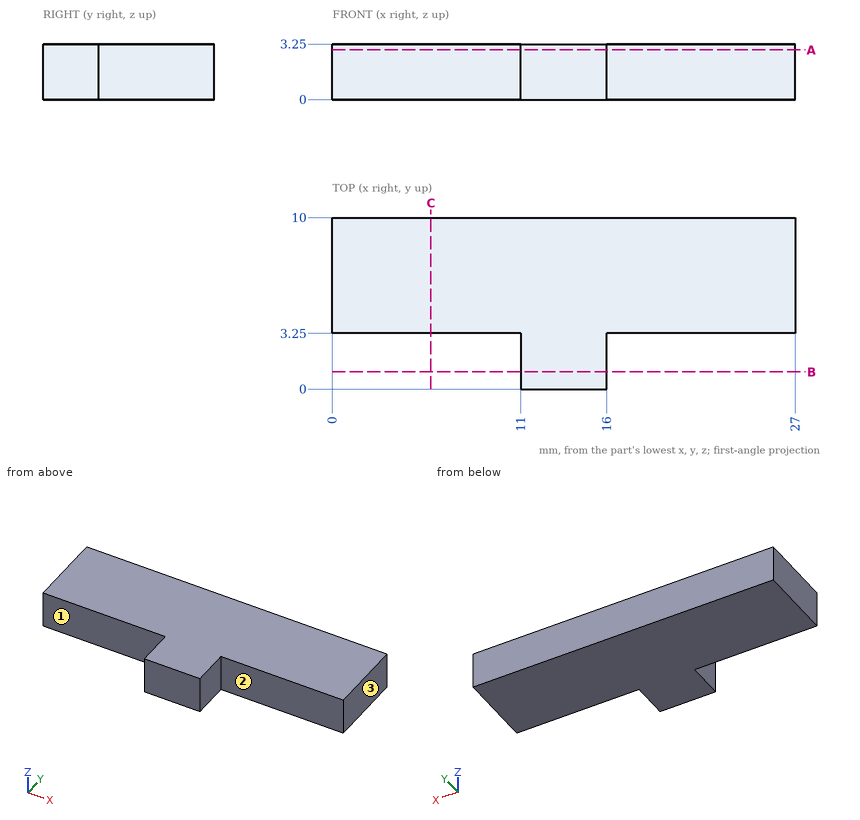
Answer from the drawing. Dimensions are ordinates in mm from the lowest x, y and z of the part. A direction names the side the tool comes from. Give positions to 0.01 mm unless a question says otherwise; leave off trailing zeros. Write each loop counter-clockwise with the first axis right and the second up, starting at its lowest first coordinate (ties: lowest second). Pieces come first, ordered by that corner, then holes. Notation, with made-up numbers: (-18.5, 32) - (9.5, 32) arc R11 ccw to (9.5, 40) - close; hole circle Ø2 at (29, 68). An arc over 180 degrees is marked (long way). Answer in a Markdown table with one row per item. Add a question column.
Item 1: Section C-C, the plane x = 5.75 is taken. Write down the section's boundary in (y, z).
Item 2: A tool of negligible diameter and unlimited length cuts with its end or side. For the marked faces 1, 2 and 3, from which of +Z, -Z, +X, -X, +Y, -Y can it reach the whole face along a straight path? Write none if from no direction.
Item 3: Section A-A, the plane z = 2.9 is taken. Write down the section's boundary in (x, y), and give its area (4 significant figures).
Item 4: Find the intervals of material crossed by L1, parallel to X at y = 0.5, z = 2; L2, parallel to Y at x = 22.5, z = 1.3, in increasing order.
Item 5: Section B-B, the plane y = 1 is taken. Write down the section's boundary in (x, z).
Item 6: Flat-ended cylindrical pins translate along their axes: P1, Ø1, axis at x = 9, y = 6.5, coming from the -Z side; P2, Ø1, axis at y = 2, z = 1.5, coming from the +X side; P3, Ø1.6, axis at x = 7.5, z = 2, coming from the -Y side. Find the tip coordinate at first contact, or state that the pin passes through.
Recorded:
| question | item | result |
|---|---|---|
| 1 | outline | (3.25, 0) - (10, 0) - (10, 3.25) - (3.25, 3.25) - close |
| 2 | face 1 | +Z, -Z, -X, -Y |
| 2 | face 2 | +Z, -Z, +X, -Y |
| 2 | face 3 | +Z, -Z, +X, +Y, -Y |
| 3 | outline | (0, 3.25) - (11, 3.25) - (11, 0) - (16, 0) - (16, 3.25) - (27, 3.25) - (27, 10) - (0, 10) - close |
| 3 | area | 198.5 mm2 |
| 4 | L1 | x = 11 to 16 |
| 4 | L2 | y = 3.25 to 10 |
| 5 | outline | (11, 0) - (16, 0) - (16, 3.25) - (11, 3.25) - close |
| 6 | P1 | stops at z = 0 |
| 6 | P2 | stops at x = 16 |
| 6 | P3 | stops at y = 3.25 |
